Here's how the part is built. I have some questions about the finished solid (model axes, mm). Face numbers are marked on the shaded views. Round coordinates to 2 decimals unless told otherwise and drop trailing zeros. Loops run counter-clockwise (first coordinate to the right, second up) from the corner with the lowest first, then second, coordinate; pieces in that order, holes last. Notation, with made-up numbers: M 50.5,55.5 L 58.5,55.5 A23 cw 58.5,66.5 Z; hole C 55.25,13 d8. An arc over 180 degrees is marked long. Use a Markdown table: item, result.
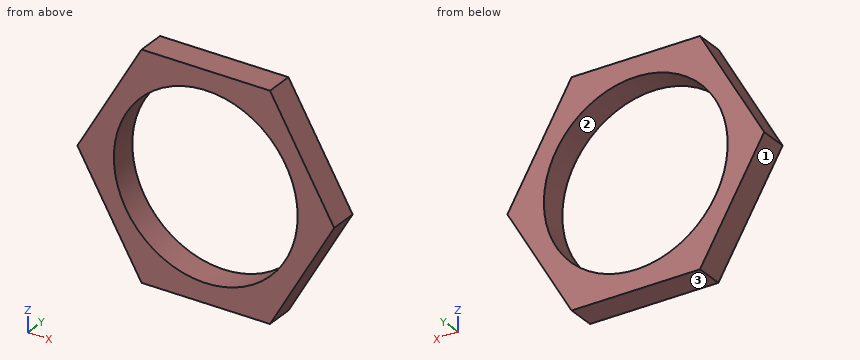
Autodesk Fusion 360 part; units mm, degrees
sketch "Sketch1" plane through (0, 0, 0) normal (0, 1, 0) x (1, 0, 0)
  circle A0 centre (0, 0) radius 7.75
  line L0 (0, 0) -> (0, -11)
  line L1 (0, 0) -> (0, 11)
  line L2 (0, -9.375) -> (-5.4127, -9.375)
  line L3 (-5.4127, -9.375) -> (-10.8253, 0)
  line L4 (-10.8253, 0) -> (-5.4127, 9.375)
  line L5 (-5.4127, 9.375) -> (0, 9.375)
  line L6 (0, 9.375) -> (5.4127, 9.375)
  line L7 (5.4127, 9.375) -> (10.8253, 0)
  line L8 (10.8253, 0) -> (5.4127, -9.375)
  line L9 (0, -9.375) -> (5.4127, -9.375)
  dimension "d1" = 15.5
  dimension "d2" = 11
  dimension "d3" = 11
  dimension "d4" = 18.75
  dimension "d5" = 9.375
  dimension "d6" = 9.375
  dimension "d7" = 9.375
  dimension "d11" = 120
  dimension "d12" = 120
  dimension "d13" = 9.375
  dimension "d14" = 9.375
extrude "Extrude1" add sketch "Sketch1" along normal blind 2.35 contours A0 L0 L1 L6 L7 L8 L9 | A0 L0 L1 L2 L3 L4 L5
equation "d3 = d2"
equation "d5 = ( 18.75 / 2 ) * 1 mm"
equation "d6 = d5"
equation "d7 = d5"
equation "d12 = d11"
equation "d13 = d5"
equation "d14 = d5"
1. I need wall thicknesses on probe 1 along Z at (x, y) = (0, 1.8) (3 decimals); probe 2 along X at (y, z) = (0.1, -5); probe 3 along X at (y, z) = (0.8, -4.5). Which ranges of each line are inside material? Lowest first, please. Write a range as from..to.
Answer sheet:
| item | result |
|---|---|
| probe 1 | -9.375..-7.75, 7.75..9.375 |
| probe 2 | -7.94..-5.92, 5.92..7.94 |
| probe 3 | -8.23..-6.31, 6.31..8.23 |
2. Imagine slicing it at C-C, the plane z = 3. Write out the boundary of the cut face in (x, y).
Answer sheet:
| item | result |
|---|---|
| outline | M -9.09,0 L -7.15,0 L -7.15,2.35 L -9.09,2.35 Z; M 7.15,0 L 9.09,0 L 9.09,2.35 L 7.15,2.35 Z |
3. Imagine slicing it at B-B, the plane x = 0. Write out the boundary of the cut face in (y, z) (3 decimals).
Answer sheet:
| item | result |
|---|---|
| outline | M 0,-9.375 L 2.35,-9.375 L 2.35,-7.75 L 0,-7.75 Z; M 0,7.75 L 2.35,7.75 L 2.35,9.375 L 0,9.375 Z |
4. For pin 1 Ø8 at (x, z) = (-7.5, 0) entering from +Y, with a flat end and sliding along its axis, tell me the tip position at first contact or that it passes through.
Answer sheet:
| item | result |
|---|---|
| pin 1 | y = 2.35 |
5. We'd pull the mould along X, two halves only. Please class the marked faces 1, 2 and 3: +X half, -X half, draft (parallel to the pull), parting line (faces both ways), or undercut.
Answer sheet:
| item | result |
|---|---|
| face 1 | -X half |
| face 2 | undercut |
| face 3 | draft |
6. Imagine slicing it at A-A, the plane y = 1.1. Write out the boundary of the cut face in (x, z) (3 decimals).
Answer sheet:
| item | result |
|---|---|
| outline | M -10.825,0 L -5.413,-9.375 L 5.413,-9.375 L 10.825,0 L 5.413,9.375 L -5.413,9.375 Z; hole C 0,0 d15.5 |
